Part model, mm, in its own coordinate system. Coordinates: 2 decimals unless noted, no trailing zeros. Write each loop counter-clockwise with the first axis right and the second up, starting at its lowest first coordinate (ties: lowest second). Pieces come first, ordered by that corner, then holes. Notation, with made-up numbers: (-14, 64.25) -> (40, 64.25) arc R21 ccw to (40, 97.25) -> close; hole circle Ø5 at (19, 61.25). An arc over 180 degrees is marked (long way). Write item = value, one per line. Start each with the question number.
Q1. Probe line 1 (X direction, y = -17, z = 2.95) (3 decimals); line 2 (Y direction, x = -6, z = 0.1); line 3 (X direction, y = -1.5, z = 0.6). List the from-to ranges inside material, lowest first.
Q2. Band-saw the part on A-A, the plane y = 14.5. List the corners of the cut face in (x, z).
Q3. Pin check, flat tips, straight feed: P1, Ø1.8, axis at x = -34.08, y = -32.64, coming from the +Z side; P2, Ø1.5, axis at x = -3.5, z = 1, coming from the -Y side; P3, Ø0.9, axis at y = -1.5, z = 1.5, coming from the +X side; P4, Ø0.9, axis at y = -15.5, z = 1.5, coming from the +X side (3 decimals). Stop position of each tip, or through.
Q4. Band-saw the part on C-C, the plane y = 3. List the corners of the cut face in (x, z), plus the area to 3 significant figures.
Q5. Band-saw the part on D-D, the plane x = -8.5. List the corners of the cut face in (y, z), plus the area to 3 significant figures.
Q6. Band-saw the part on B-B, the plane x = 42. List the corners of the cut face in (y, z), plus the area to 3 significant figures.
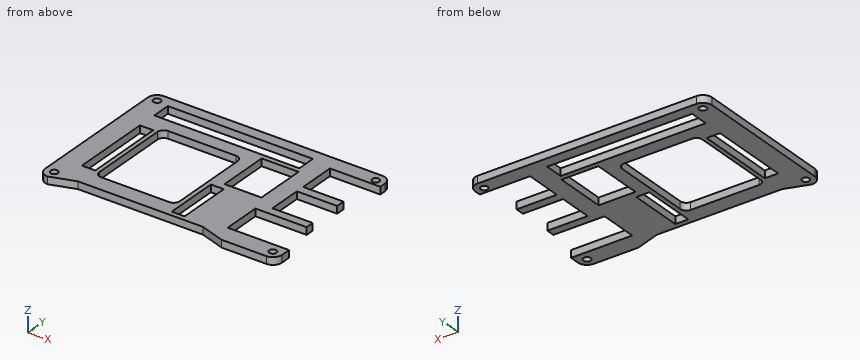
from build123d import *

# Parameters (mm, degrees)
SKETCH1_R           = 1.3462
SKETCH1_W           = 5.4034
SKETCH1_H           = 22.6066
SKETCH1_W_2         = 60.6932
SKETCH1_H_2         = 7.81
SKETCH1_W_3         = 15.431
SKETCH1_H_3         = 21.4039
SKETCH1_W_4         = 31.9679
SKETCH1_H_4         = 18.2371
SKETCH1_W_5         = 5.588
SKETCH1_H_5         = 33.5001
BOSS_EXTRUDE1_DEPTH = 3.048
SKETCH2_W           = 33.5789
SKETCH2_H           = 38.5801
CUT_EXTRUDE1_DEPTH  = 4.048
FILLET1_R           = 2.54
SKETCH3_R           = 1.524
CUT_EXTRUDE2_DEPTH  = 4.048


with BuildPart() as part:
    # Sketch1 → Boss-Extrude1 (new body)
    with BuildSketch(Plane.XY):
        with BuildLine():
            Line((61.214907375, 24.068294304), (40.134807375, 24.068294304))
            Line((40.134807375, 24.068294304), (40.134807375, 8.658194304))
            Line((40.134807375, 8.658194304), (56.975007375, 8.658194304))
            Line((56.975007375, 8.658194304), (56.975007375, 4.997894304))
            Line((56.975007375, 4.997894304), (40.134807375, 4.997894304))
            Line((40.134807375, 4.997894304), (40.134807375, -9.121805696))
            Line((40.134807375, -9.121805696), (56.975007375, -9.121805696))
            Line((56.975007375, -9.121805696), (56.975007375, -12.628005696))
            Line((56.975007375, -12.628005696), (35.575007375, -12.628005696))
            Line((35.575007375, -12.628005696), (35.575007375, -28.627805696))
            Line((35.575007375, -28.627805696), (61.214907375, -28.627805696))
            Line((61.214907375, -28.627805696), (61.214907375, -32.613401529))
            ThreePointArc((61.214907375, -32.613401529), (60.108826144, -35.325305244), (57.405007375, -36.451005696))
            Line((57.405007375, -36.451005696), (38.714307375, -36.451005696))
            Line((38.714307375, -36.451005696), (28.474307375, -33.084405696))
            Line((28.474307375, -33.084405696), (-23.844892625, -33.084405696))
            Line((-23.844892625, -33.084405696), (-34.084892625, -36.451005696))
            ThreePointArc((-34.084892625, -36.451005696), (-36.778969461, -35.335082532), (-37.894892625, -32.641005696))
            Line((-37.894892625, -32.641005696), (-37.894892625, 26.697694304))
            ThreePointArc((-37.894892625, 26.697694304), (-36.778969461, 29.391771141), (-34.084892625, 30.507694304))
            Line((-34.084892625, 30.507694304), (57.404932375, 30.507694304))
            ThreePointArc((57.404932375, 30.507694304), (60.103884597, 29.386886916), (61.214907375, 26.683892153))
            Line((61.214907375, 26.683892153), (61.214907375, 24.068294304))
        make_face()
        with Locations((57.404932375, 26.697694304)):
            Circle(SKETCH1_R, mode=Mode.SUBTRACT)
        with Locations((57.405007375, -32.641005696)):
            Circle(SKETCH1_R, mode=Mode.SUBTRACT)
        with Locations((-34.084892625, -32.641005696)):
            Circle(SKETCH1_R, mode=Mode.SUBTRACT)
        with Locations((-34.084892625, 26.697694304)):
            Circle(SKETCH1_R, mode=Mode.SUBTRACT)
        with Locations((16.546707375, -19.663505696)):
            Rectangle(SKETCH1_W, SKETCH1_H, mode=Mode.SUBTRACT)
        with Locations((1.341707375, 21.991994304)):
            Rectangle(SKETCH1_W_2, SKETCH1_H_2, mode=Mode.SUBTRACT)
        with Locations((25.156507375, 5.270444304)):
            Rectangle(SKETCH1_W_3, SKETCH1_H_3, mode=Mode.SUBTRACT)
        with Locations((-5.654942625, 1.475544304)):
            Rectangle(SKETCH1_W_4, SKETCH1_H_4, mode=Mode.SUBTRACT)
        with Locations((-26.210892625, -6.948855696)):
            Rectangle(SKETCH1_W_5, SKETCH1_H_5, mode=Mode.SUBTRACT)
    extrude(amount=BOSS_EXTRUDE1_DEPTH)

    # Sketch2 → Cut-Extrude1 (cut, through all)
    with BuildSketch(Plane.XY.offset(3.048)):
        with Locations((-4.849442625, -6.948855696)):
            Rectangle(SKETCH2_W, SKETCH2_H)
    extrude(amount=-CUT_EXTRUDE1_DEPTH, mode=Mode.SUBTRACT)

    # Fillet1
    fillet1_edges = [part.edges().sort_by_distance(p)[0] for p in [
        (-21.638892625, -26.238905696, 1.524),
        (11.940007375, 12.341194304, 1.524),
        (11.940007375, -26.238905696, 1.524),
        (-21.638892625, 12.341194304, 1.524),
    ]]
    fillet(fillet1_edges, radius=FILLET1_R)

    # Sketch3 → Cut-Extrude2 (cut, through all)
    with BuildSketch(Plane.XY.offset(3.048)):
        with Locations((-34.084892625, 26.697694304)):
            Circle(SKETCH3_R)
        with Locations((57.404932375, 26.697694304)):
            Circle(SKETCH3_R)
        with Locations((57.405007375, -32.641005696)):
            Circle(SKETCH3_R)
        with Locations((-34.084892625, -32.641005696)):
            Circle(SKETCH3_R)
    extrude(amount=-CUT_EXTRUDE2_DEPTH, mode=Mode.SUBTRACT)


solid = part.part
Ans:
q1.line_1 = -37.895 to -29.005, -23.417 to -21.639, 11.94 to 13.845, 19.248 to 35.575
q1.line_2 = -33.08 to -26.24, 12.34 to 18.09, 25.9 to 30.51
q1.line_3 = -37.89 to -29, -23.42 to -21.64, 11.94 to 17.44, 32.87 to 40.13
q2.outline = (-37.89, 0) -> (17.44, 0) -> (17.44, 3.05) -> (-37.89, 3.05) -> close; (32.87, 0) -> (40.13, 0) -> (40.13, 3.05) -> (32.87, 3.05) -> close
q3.P1 = through
q3.P2 = -33.08
q3.P3 = 40.13
q3.P4 = 35.575
q4.outline = (-37.89, 0) -> (-29, 0) -> (-29, 3.05) -> (-37.89, 3.05) -> close; (-23.42, 0) -> (-21.64, 0) -> (-21.64, 3.05) -> (-23.42, 3.05) -> close; (11.94, 0) -> (17.44, 0) -> (17.44, 3.05) -> (11.94, 3.05) -> close; (32.87, 0) -> (40.13, 0) -> (40.13, 3.05) -> (32.87, 3.05) -> close
q4.area = 71.4 mm2
q5.outline = (-33.08, 0) -> (-26.24, 0) -> (-26.24, 3.05) -> (-33.08, 3.05) -> close; (12.34, 0) -> (18.09, 0) -> (18.09, 3.05) -> (12.34, 3.05) -> close; (25.9, 0) -> (30.51, 0) -> (30.51, 3.05) -> (25.9, 3.05) -> close
q5.area = 52.4 mm2
q6.outline = (-36.45, 0) -> (-28.63, 0) -> (-28.63, 3.05) -> (-36.45, 3.05) -> close; (-12.63, 0) -> (-9.12, 0) -> (-9.12, 3.05) -> (-12.63, 3.05) -> close; (5, 0) -> (8.66, 0) -> (8.66, 3.05) -> (5, 3.05) -> close; (24.07, 0) -> (30.51, 0) -> (30.51, 3.05) -> (24.07, 3.05) -> close
q6.area = 65.3 mm2
